Source: three-view drawing plus pictorial views. Frame: mm from the lowest corner of the part. Give positions to 0.01 mm unless a question says otherwise; leave off trailing zeros. Loops run counter-clockwise (first coordinate to the right, second up) from the corner with the lowest first, then second, coordinate; pieces in that order, holes last. Notation, with made-up numbers: (62.5, 17.5) - (86.5, 17.5) arc R18 ccw to (86.5, 43.5) - close; hole circle Ø1 at (77.25, 78). An arc over 180 degrees is marked (long way). Answer as a JSON object with one key per item and string values.
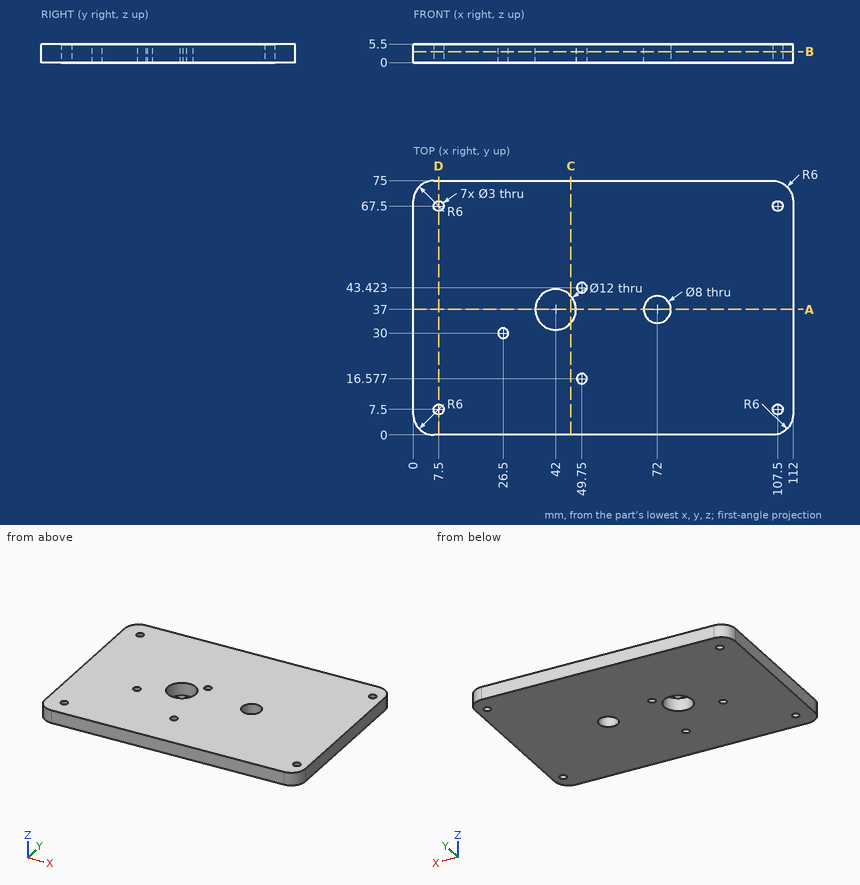
Item 1: Cut plane B-B (z = 3.25). Give the number of separate pieces and of enclosed holes in the cut face, then the cut area to 3 significant figures.
Geometry check:
{"separate pieces": "1", "enclosed holes": "9", "area": "8,160 mm2"}
Item 2: Cut plane A-A (y = 37). Return loops of the section in (x, z).
Geometry check:
{"outline": "(0, 0) - (36, 0) - (36, 5.5) - (0, 5.5) - close; (48, 0) - (68, 0) - (68, 5.5) - (48, 5.5) - close; (76, 0) - (112, 0) - (112, 5.5) - (76, 5.5) - close"}
Item 3: Cut plane C-C (x = 46.5). Return loops of the section in (y, z), then the cut area to 3 significant figures.
Geometry check:
{"outline": "(0, 0) - (33.03, 0) - (33.03, 5.5) - (0, 5.5) - close; (40.97, 0) - (75, 0) - (75, 5.5) - (40.97, 5.5) - close", "area": "369 mm2"}
Item 4: Cut plane D-D (x = 7.5). Return loops of the section in (y, z).
Geometry check:
{"outline": "(0, 0) - (6, 0) - (6, 5.5) - (0, 5.5) - close; (9, 0) - (66, 0) - (66, 5.5) - (9, 5.5) - close; (69, 0) - (75, 0) - (75, 5.5) - (69, 5.5) - close"}
Item 5: Material intervals for line 1 (X direction, y = 7.5, z = 3.95); line 2 (Y direction, x = 49.75, z = 3.4); line 3 (Y direction, x = 26.5, z = 2.2), sorted ascending. Write a range as [from, to].
Geometry check:
{"line 1": "x = [0, 6], [9, 106], [109, 112]", "line 2": "y = [0, 15.08], [18.08, 41.92], [44.92, 75]", "line 3": "y = [0, 28.5], [31.5, 75]"}
